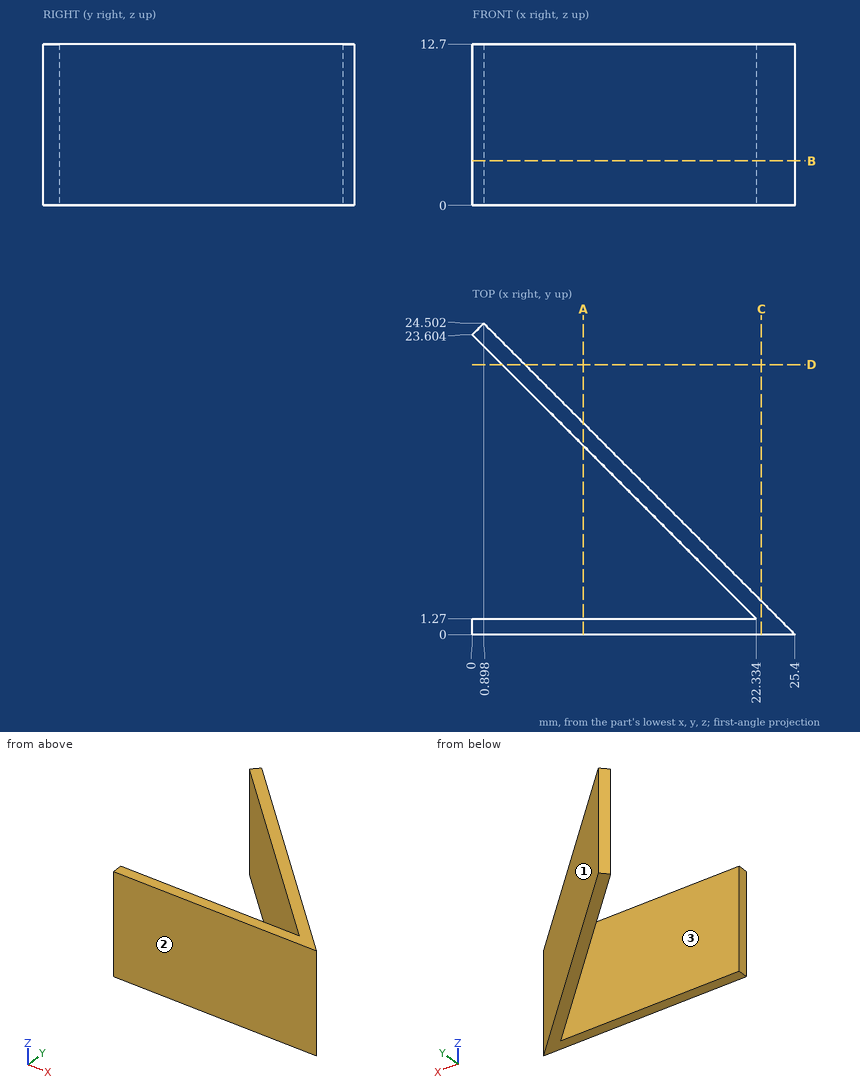
Check sheet for the drawn part. Datum: minimum x, y, z corner. Units: mm. Coordinates: 2 decimals unless noted, no trailing zeros. Write each loop counter-clockwise with the first axis right and the second up, starting at its lowest first coordinate (ties: lowest second). Pieces come first, ordered by that corner, then holes. Notation, with made-up numbers: M 40.25,-39 L 55.25,-39 A15 cw 55.25,-22 Z; hole C -19,44.5 d3. An arc over 180 degrees is marked long. Use a Markdown table: item, result.
Q1. Thickness scan on line 1 (Y direction, x = 19, z = 9); line 2 (Y direction, x = 17, z = 12.25); line 3 (X direction, y = 23.25, z = 11). Record the ranges inside material, lowest first.
Reply:
| item | result |
|---|---|
| line 1 | y = 0 to 1.27, 4.6 to 6.4 |
| line 2 | y = 0 to 1.27, 6.6 to 8.4 |
| line 3 | x = 0.35 to 2.15 |
Q2. Draft check along Y on the marked faces 1, 2 and 3. Enter one of: +Y half, -Y half, draft (parallel to the pull), parting line (faces both ways), or undercut.
Reply:
| item | result |
|---|---|
| face 1 | +Y half |
| face 2 | -Y half |
| face 3 | undercut |
Q3. Sectioned sample at A-A, the plane x = 8.75. Record the boundary of the cut face in (y, z).
Reply:
| item | result |
|---|---|
| outline | M 0,0 L 1.27,0 L 1.27,12.7 L 0,12.7 Z; M 14.85,0 L 16.65,0 L 16.65,12.7 L 14.85,12.7 Z |
Q4. Sectioned sample at D-D, the plane y = 21.25. Record the boundary of the cut face in (x, z).
Reply:
| item | result |
|---|---|
| outline | M 2.35,0 L 4.15,0 L 4.15,12.7 L 2.35,12.7 Z |
Q5. Sectioned sample at B-B, the plane z = 3.5. Record the boundary of the cut face in (x, y).
Reply:
| item | result |
|---|---|
| outline | M 0,0 L 25.4,0 L 0.9,24.5 L 0,23.6 L 22.33,1.27 L 0,1.27 Z |
Q6. Go/stop test with flat-tipped pins: P1, Ø1.5, axis at y = 9.5, z = 6, coming from the -X side; P2, Ø1, axis at x = 7, z = 7, coming from the +Y side; P3, Ø2, axis at y = 5.5, z = 4, coming from the +X side. Record where each tip stops, or that it passes through.
Reply:
| item | result |
|---|---|
| P1 | stops at x = 13.35 |
| P2 | stops at y = 18.9 |
| P3 | stops at x = 20.9 |
Q7. Sectioned sample at C-C, the plane x = 22.75. Record the boundary of the cut face in (y, z).
Reply:
| item | result |
|---|---|
| outline | M 0,0 L 2.65,0 L 2.65,12.7 L 0,12.7 Z |
